Can you work these out from the drawing? Everything is in mm from the part's minimum corner. A direction names the side the tool comes from. Round coordinates to 2 decimals unless told otherwise and drop trailing zeros. Order: outer loops, then holes, each group sorted by start corner. A loop starts at its lowest first (then second) coordinate and runs counter-clockwise, first axis right, second up. Notation, with made-up numbers: (-12, -36.5) -> (24, -36.5) arc R29 cw to (24, -2.5) -> close; hole circle Ø10 at (46, 6.25). An arc over 180 degrees is marked (long way). One line per item, written item: value.
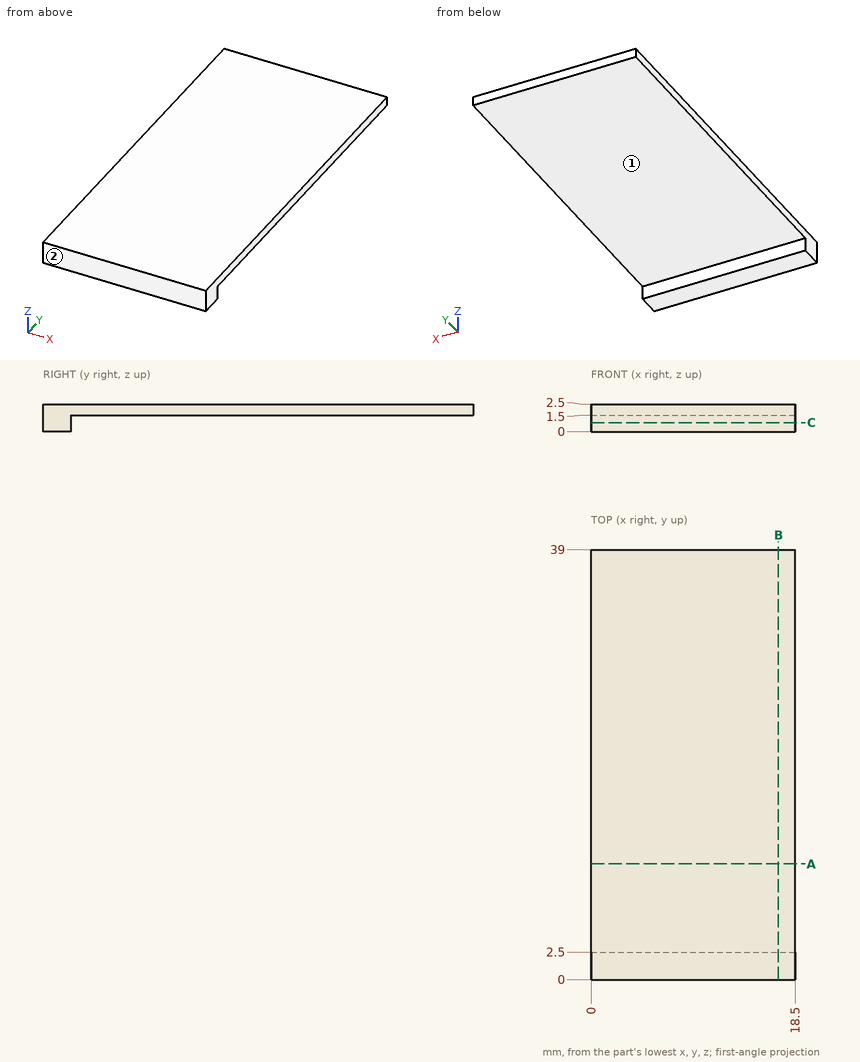
Q1. I want a section at B-B on x = 17. Write out the boundary of the cut face in (y, z).
Answers:
outline: (0, 0) -> (2.5, 0) -> (2.5, 1.5) -> (39, 1.5) -> (39, 2.5) -> (0, 2.5) -> close
Q2. I need wall thicknesses on line 1 along Y through (x, z) = (9.5, 0.45); line 2 along Z through (x, y) = (3.25, 19). Which ranges of each line are inside material? Lowest first, please.
Answers:
line 1: 0 to 2.5
line 2: 1.5 to 2.5
Q3. For P1, Ø1, axis at x = 8, z = 0.5, coming from the +Y side; P2, Ø9, axis at x = 13.5, y = 30, coming from the -Z side, each with a flat end and sliding along its axis, tell me the tip position at first contact or that it passes through.
Answers:
P1: y = 2.5
P2: z = 1.5
Q4. Which directions (+Z, -Z, +X, -X, +Y, -Y) give clear straight access to the entire face, cutting with the end or side of a thin tool? Please do the marked faces 1 and 2.
Answers:
face 1: -Z, +X, -X, +Y
face 2: +Z, -Z, +X, -X, -Y
Q5. I want a section at C-C on z = 0.8. Write out the boundary of the cut face in (x, y).
Answers:
outline: (0, 0) -> (18.5, 0) -> (18.5, 2.5) -> (0, 2.5) -> close
Q6. I want a section at A-A on y = 10.5. Write out the boundary of the cut face in (x, z).
Answers:
outline: (0, 1.5) -> (18.5, 1.5) -> (18.5, 2.5) -> (0, 2.5) -> close
